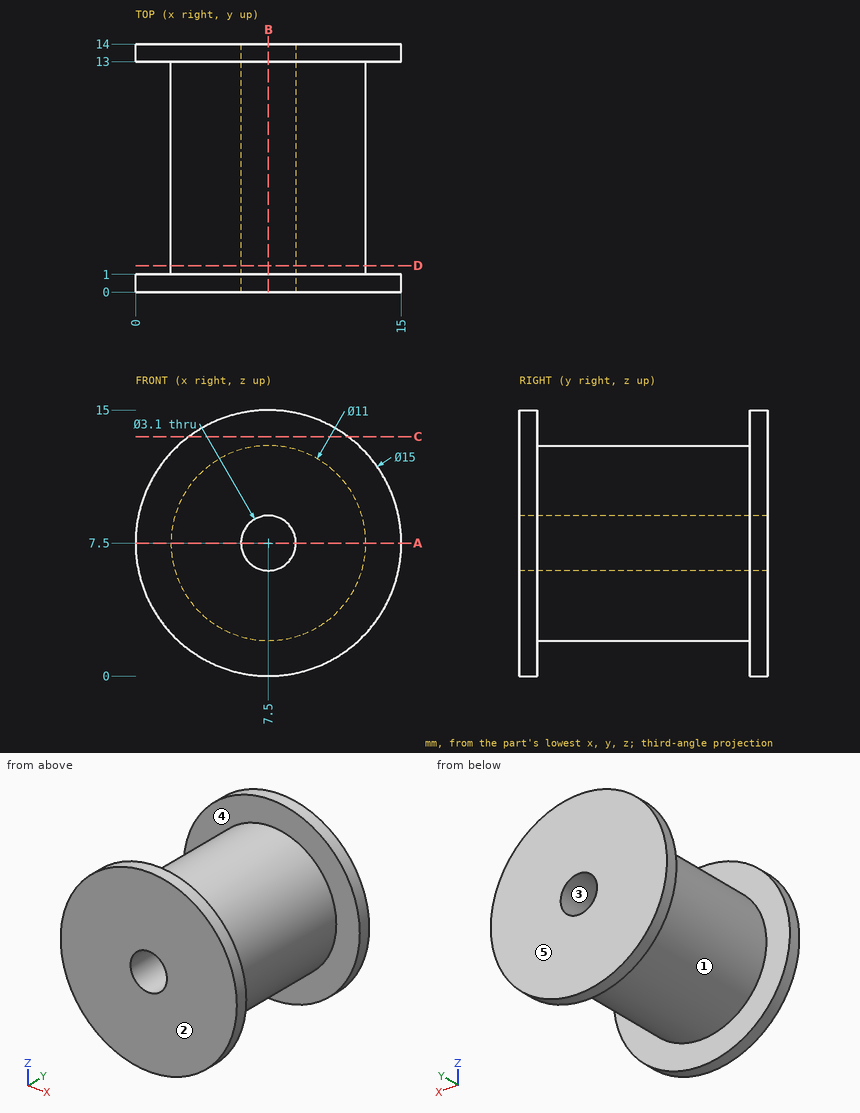
Input: dimensioned drawing with shaded views. Units: mm. Origin: part minimum x, y, z. A direction names the side the tool comes from. Give positions to 0.01 mm unless a question says otherwise; leave off trailing zeros. Write each loop counter-clockwise with the first axis right and the second up, starting at its lowest first coordinate (ties: lowest second). Pieces come first, ordered by that corner, then holes. Notation, with made-up numbers: (39.5, -9) -> (70.5, -9) arc R11 cw to (70.5, 0) -> close; hole circle Ø10 at (66, 89). An arc over 180 degrees is marked (long way). Return JSON: item names as keys, results as strings. Group by question number.
1. Mould query, pull axis X, two halves, no side actions, for the marked faces 1, 2 and 3. Classes: +X half, -X half, draft (parallel to the pull), parting line (faces both ways), or undercut.
2. Section B-B, the plane x = 7.5. Output: boundary loops of the cut face in (y, z), then the cut area to 3 significant figures.
3. Section A-A, the plane z = 7.5. Output: boundary loops of the cut face in (x, y), then the cut area to 3 significant figures.
4. Section D-D, the plane y = 1.5. Output: boundary loops of the cut face in (x, z), then the cut area to 3 significant figures.
5. Material intervals for line 1 (Z direction, x = 7.5, y = 9); line 2 (Y direction, x = 5, z = 12.5); line 3 (X direction, y = 7.25, z = 8.75), sorted ascending. Write a range as from..to.
6. Access query for the marked faces 4 and 5. Directions: +Z, -Z, +X, -X, +Y, -Y. A direction counts if a zero-diameter tool reaches every point of the face in a straight line with its end or side. Return the directions, or none.
7. Section C-C, the plane z = 13.5. Output: boundary loops of the cut face in (x, y), then the cut area to 3 significant figures.
8. Pin query (flat end, axial travel): pin 1 Ø8 at (x, y) = (9.5, 7.5) entering from -Z; pin 2 Ø2 at (x, y) = (5, 2.5) entering from -Z; pin 3 Ø6 at (y, z) = (8.5, 10.5) entering from +X. Return the tip coordinate at first contact, or that it passes through.
Determined:
{
 "1": {"face 1": "parting line", "face 2": "draft", "face 3": "undercut"},
 "2": {"outline": "(0, 0) -> (1, 0) -> (1, 2) -> (13, 2) -> (13, 0) -> (14, 0) -> (14, 5.95) -> (0, 5.95) -> close; (0, 9.05) -> (14, 9.05) -> (14, 15) -> (13, 15) -> (13, 13) -> (1, 13) -> (1, 15) -> (0, 15) -> close", "area": "119 mm2"},
 "3": {"outline": "(0, 0) -> (5.95, 0) -> (5.95, 14) -> (0, 14) -> (0, 13) -> (2, 13) -> (2, 1) -> (0, 1) -> close; (9.05, 0) -> (15, 0) -> (15, 1) -> (13, 1) -> (13, 13) -> (15, 13) -> (15, 14) -> (9.05, 14) -> close", "area": "119 mm2"},
 "4": {"outline": "circle Ø11 at (7.5, 7.5); hole circle Ø3.1 at (7.5, 7.5)", "area": "87.5 mm2"},
 "5": {"line 1": "z = 2..5.95, 9.05..13", "line 2": "y = 0..1, 13..14", "line 3": "x = 2.14..6.58, 8.42..12.86"},
 "6": {"face 4": "none", "face 5": "+Z, -Z, +X, -X, +Y"},
 "7": {"outline": "(3, 0) -> (12, 0) -> (12, 1) -> (3, 1) -> close; (3, 13) -> (12, 13) -> (12, 14) -> (3, 14) -> close", "area": "18.0 mm2"},
 "8": {"pin 1": "stops at z = 2", "pin 2": "stops at z = 2.21", "pin 3": "stops at x = 13"}
}
